The drawing under review shows one solid part. Ordinate dimensions are in mm from its lowest x, y, z. A direction names the side the tool comes from. Coordinates: 2 decimals unless noted, no trailing zeros. Loops run counter-clockwise (first coordinate to the right, second up) from the corner with the lowest first, then second, coordinate; pieces in that order, holes last. Notation, with made-up numbers: M -8.75,42.5 L 34.25,42.5 A19 ccw 34.25,61.5 Z; hole C -6,56.25 d3. An arc over 180 degrees is marked long. Answer as CSV lines item,"result". Start each with the question number.
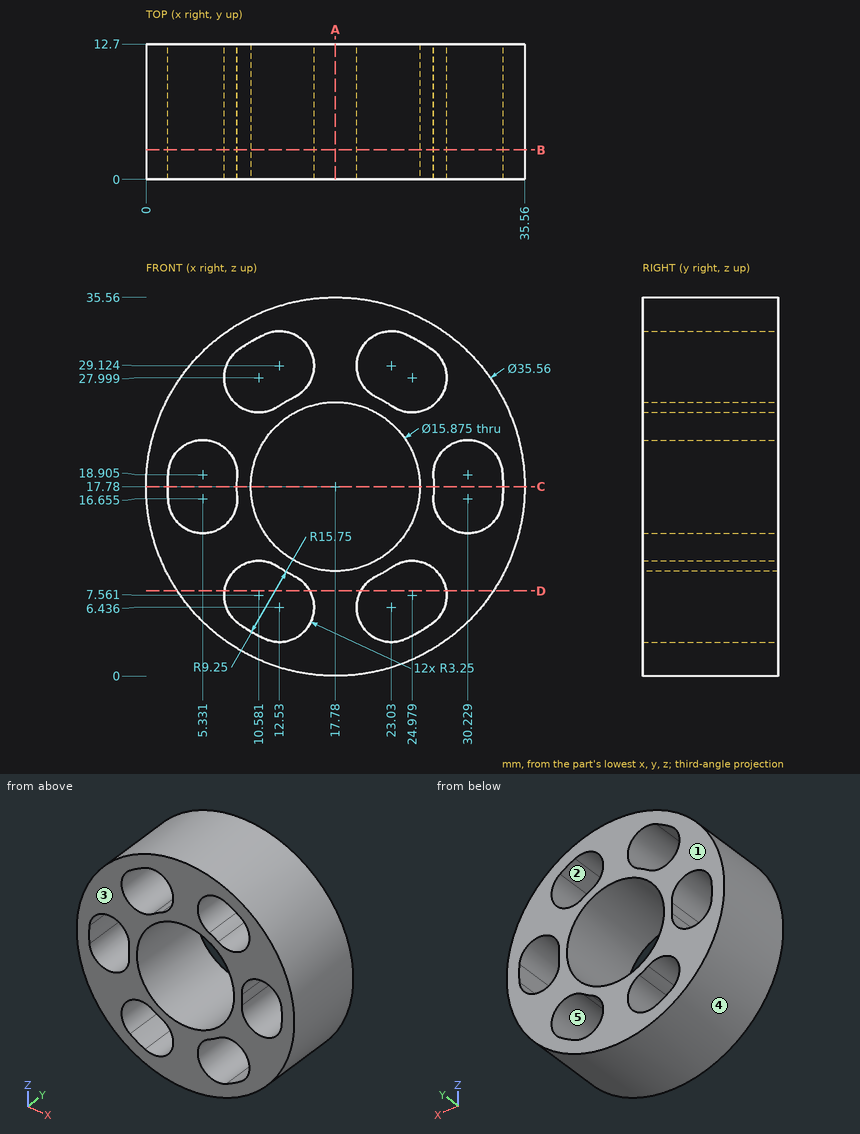
Item 1: For line 1 along X through (y, z) = (3.5, 17.78); line 2 along X through (y, z) = (5.5, 8); line 3 along X through (y, z) = (7.75, 27.5) (1 decimal), list the stretches that pass through material, from the lowest coordinate up. Write a range as from..to.
Item 2: For the marked faces 1 and 2, list the 3-axis set-ups (+Z, -Z, +X, -X, +Y, -Y) from which the entire face can be reached by the end or side of a thin tool; tool diameter is ignored.
Item 3: Mouldability with a two-part tool opening along X and no side actions: class the marked faces 3, 4 and 5 as released by +X, released by -X, zero draft, split by the parting line, or undercut.
Item 4: Add section A-A (x = 17.78). Give the boundary of the cut face in (y, z).
Item 5: For pin 1 (3 mm diameter, centred on x = 4, y = 9, fed in from +Z); pin 2 (5 mm diameter, centred on x = 5.5, y = 4.5, fed in from +Z); pin 3 (2 mm diameter, centred on x = 14, y = 9.5, fed in from +Z), all flat-tipped, find the tip position at first contact; note any pin that passes through.
Item 6: Add section B-B (y = 2.75). Give the number of separate pieces and of enclosed holes in the cut face, plus the area to 3 significant figures.
Item 7: Add section D-D (z = 8). Give the boundary of the cut face in (x, y).
Item 8: Add section C-C (z = 17.78). Give the boundary of the cut face in (x, y).
Response:
1,line 1,"0..2.03, 8.53..9.84, 25.72..27.03, 33.53..35.56"
1,line 2,"2.93..7.36, 15.38..20.18, 28.2..32.63"
1,line 3,"2.9..7.4, 15.3..20.2, 28.2..32.7"
2,face 1,"+Z, -Z, +X, -X, +Y"
2,face 2,"+Y, -Y"
3,face 3,"zero draft"
3,face 4,"split by the parting line"
3,face 5,"undercut"
4,outline,"M 0,0 L 12.7,0 L 12.7,9.84 L 0,9.84 Z; M 0,25.72 L 12.7,25.72 L 12.7,35.56 L 0,35.56 Z"
5,pin 1,"z = 30.64"
5,pin 2,"z = 32.63"
5,pin 3,"z = 35.34"
6,separate pieces,"1"
6,enclosed holes,"7"
6,area,"508 mm²"
7,outline,"M 2.93,0 L 7.36,0 L 7.36,12.7 L 2.93,12.7 Z; M 15.38,0 L 20.18,0 L 20.18,12.7 L 15.38,12.7 Z; M 28.2,0 L 32.63,0 L 32.63,12.7 L 28.2,12.7 Z"
8,outline,"M 0,0 L 2.03,0 L 2.03,12.7 L 0,12.7 Z; M 8.53,0 L 9.84,0 L 9.84,12.7 L 8.53,12.7 Z; M 25.72,0 L 27.03,0 L 27.03,12.7 L 25.72,12.7 Z; M 33.53,0 L 35.56,0 L 35.56,12.7 L 33.53,12.7 Z"
